from build123d import *

# Parameters (mm, degrees)
F1_DEPTH = 3
F2_R     = 1.25
F3_DEPTH = 10
F4_R     = 1
F5_DEPTH = 25
F6_W     = 1
F6_H     = 75
F7_DEPTH = 1


with BuildPart() as f1:
    # F0 (on Top) → F1 (new body)
    with BuildSketch(Plane.XY):
        with BuildLine():
            ThreePointArc((8.915987, -1.226854), (8.978972, -0.614863), (9, 0))
            ThreePointArc((9, 0), (8.978972, 0.614863), (8.915987, 1.226854))
            ThreePointArc((8.915987, 1.226854), (8.559509, 2.781153), (7.934312, 4.24814))
            ThreePointArc((7.934312, 4.24814), (7.281153, 5.290067), (6.492059, 6.233231))
            ThreePointArc((6.492059, 6.233231), (5.290067, 7.281153), (3.921999, 8.100489))
            ThreePointArc((3.921999, 8.100489), (2.781153, 8.559509), (1.588385, 8.858726))
            ThreePointArc((1.588385, 8.858726), (0, 9), (-1.588385, 8.858726))
            ThreePointArc((-1.588385, 8.858726), (-2.781153, 8.559509), (-3.921999, 8.100489))
            ThreePointArc((-3.921999, 8.100489), (-5.290067, 7.281153), (-6.492059, 6.233231))
            ThreePointArc((-6.492059, 6.233231), (-7.281153, 5.290067), (-7.934312, 4.24814))
            ThreePointArc((-7.934312, 4.24814), (-8.559509, 2.781153), (-8.915987, 1.226854))
            ThreePointArc((-8.915987, 1.226854), (-9, 0), (-8.915987, -1.226854))
            ThreePointArc((-8.915987, -1.226854), (-8.559509, -2.781153), (-7.934312, -4.24814))
            ThreePointArc((-7.934312, -4.24814), (-7.281153, -5.290067), (-6.492059, -6.233231))
            ThreePointArc((-6.492059, -6.233231), (-5.290067, -7.281153), (-3.921999, -8.100489))
            ThreePointArc((-3.921999, -8.100489), (-2.781153, -8.559509), (-1.588385, -8.858726))
            ThreePointArc((-1.588385, -8.858726), (0, -9), (1.588385, -8.858726))
            ThreePointArc((1.588385, -8.858726), (2.781153, -8.559509), (3.921999, -8.100489))
            ThreePointArc((3.921999, -8.100489), (5.290067, -7.281153), (6.492059, -6.233231))
            ThreePointArc((6.492059, -6.233231), (7.281153, -5.290067), (7.934312, -4.24814))
            ThreePointArc((7.934312, -4.24814), (8.559509, -2.781153), (8.915987, -1.226854))
        make_face()
        with BuildLine():
            ThreePointArc((7.934312, 4.24814), (8.559509, 2.781153), (8.915987, 1.226854))
            ThreePointArc((8.915987, 1.226854), (10.16558, 1.771623), (11.246167, 2.602639))
            Line((11.246167, 2.602639), (10.93715, 3.553695))
            Line((10.93715, 3.553695), (10.628133, 4.504752))
            ThreePointArc((10.628133, 4.504752), (9.265461, 4.541905), (7.934312, 4.24814))
        make_face()
        with BuildLine():
            ThreePointArc((11.246167, -2.602639), (10.16558, -1.771623), (8.915987, -1.226854))
            ThreePointArc((8.915987, -1.226854), (8.559509, -2.781153), (7.934312, -4.24814))
            ThreePointArc((7.934312, -4.24814), (9.265461, -4.541905), (10.628133, -4.504752))
            Line((10.628133, -4.504752), (10.93715, -3.553695))
            Line((10.93715, -3.553695), (11.246167, -2.602639))
        make_face()
        with BuildLine():
            ThreePointArc((3.921999, 8.100489), (5.290067, 7.281153), (6.492059, 6.233231))
            ThreePointArc((6.492059, 6.233231), (7.182793, 7.408451), (7.568547, 8.71591))
            Line((7.568547, 8.71591), (6.75953, 9.303695))
            Line((6.75953, 9.303695), (5.950513, 9.891481))
            ThreePointArc((5.950513, 9.891481), (4.826251, 9.120579), (3.921999, 8.100489))
        make_face()
        with BuildLine():
            ThreePointArc((7.568547, -8.71591), (7.182793, -7.408451), (6.492059, -6.233231))
            ThreePointArc((6.492059, -6.233231), (5.290067, -7.281153), (3.921999, -8.100489))
            ThreePointArc((3.921999, -8.100489), (4.826251, -9.120579), (5.950513, -9.891481))
            Line((5.950513, -9.891481), (6.75953, -9.303695))
            Line((6.75953, -9.303695), (7.568547, -8.71591))
        make_face()
        with BuildLine():
            ThreePointArc((-1.588385, 8.858726), (0, 9), (1.588385, 8.858726))
            ThreePointArc((1.588385, 8.858726), (1.456423, 10.215503), (1, 11.5))
            Line((1, 11.5), (0, 11.5))
            Line((0, 11.5), (-1, 11.5))
            ThreePointArc((-1, 11.5), (-1.456423, 10.215503), (-1.588385, 8.858726))
        make_face()
        with BuildLine():
            ThreePointArc((1, -11.5), (1.456423, -10.215503), (1.588385, -8.858726))
            ThreePointArc((1.588385, -8.858726), (0, -9), (-1.588385, -8.858726))
            ThreePointArc((-1.588385, -8.858726), (-1.456423, -10.215503), (-1, -11.5))
            Line((-1, -11.5), (0, -11.5))
            Line((0, -11.5), (1, -11.5))
        make_face()
        with BuildLine():
            ThreePointArc((-6.492059, 6.233231), (-5.290067, 7.281153), (-3.921999, 8.100489))
            ThreePointArc((-3.921999, 8.100489), (-4.826251, 9.120579), (-5.950513, 9.891481))
            Line((-5.950513, 9.891481), (-6.75953, 9.303695))
            Line((-6.75953, 9.303695), (-7.568547, 8.71591))
            ThreePointArc((-7.568547, 8.71591), (-7.182793, 7.408451), (-6.492059, 6.233231))
        make_face()
        with BuildLine():
            ThreePointArc((-5.950513, -9.891481), (-4.826251, -9.120579), (-3.921999, -8.100489))
            ThreePointArc((-3.921999, -8.100489), (-5.290067, -7.281153), (-6.492059, -6.233231))
            ThreePointArc((-6.492059, -6.233231), (-7.182793, -7.408451), (-7.568547, -8.71591))
            Line((-7.568547, -8.71591), (-6.75953, -9.303695))
            Line((-6.75953, -9.303695), (-5.950513, -9.891481))
        make_face()
        with BuildLine():
            ThreePointArc((-8.915987, 1.226854), (-8.559509, 2.781153), (-7.934312, 4.24814))
            ThreePointArc((-7.934312, 4.24814), (-9.265461, 4.541905), (-10.628133, 4.504752))
            Line((-10.628133, 4.504752), (-10.93715, 3.553695))
            Line((-10.93715, 3.553695), (-11.246167, 2.602639))
            ThreePointArc((-11.246167, 2.602639), (-10.16558, 1.771623), (-8.915987, 1.226854))
        make_face()
        with BuildLine():
            ThreePointArc((-10.628133, -4.504752), (-9.265461, -4.541905), (-7.934312, -4.24814))
            ThreePointArc((-7.934312, -4.24814), (-8.559509, -2.781153), (-8.915987, -1.226854))
            ThreePointArc((-8.915987, -1.226854), (-10.16558, -1.771623), (-11.246167, -2.602639))
            Line((-11.246167, -2.602639), (-10.93715, -3.553695))
            Line((-10.93715, -3.553695), (-10.628133, -4.504752))
        make_face()
    extrude(amount=F1_DEPTH)

    # F2 (on face) → F3 (join)
    with BuildSketch(Plane.XY.offset(3)):
        Circle(F2_R)
    extrude(amount=F3_DEPTH)

    # F4 (on face) → F5 (cut)
    with BuildSketch(Plane.XY.offset(13)):
        Circle(F4_R)
    extrude(amount=-F5_DEPTH, mode=Mode.SUBTRACT)

    # F6 (on face) → F7 (join)
    with BuildSketch(Plane.XY.offset(13)):
        with BuildLine():
            ThreePointArc((-1, 0.75), (-0.559017, 1.118034), (0, 1.25))
            Line((0, 1.25), (-1, 1.25))
            Line((-1, 1.25), (-1, 0.75))
        make_face()
        with Locations((-0.5, 38.75)):
            Rectangle(F6_W, F6_H)
        with Locations((0.5, 38.75)):
            Rectangle(F6_W, F6_H)
        with BuildLine():
            Line((1, 1.25), (0, 1.25))
            ThreePointArc((0, 1.25), (0.559017, 1.118034), (1, 0.75))
            Line((1, 0.75), (1, 1.25))
        make_face()
    extrude(amount=-F7_DEPTH)


solid = f1.part
Read the model definition and answer for the solid it produces. Units are mm, in the model's axes. A direction names the side the tool comes from. Round coordinates to 2 decimals unless told otherwise and drop trailing zeros. Write each loop counter-clockwise with the first axis right and the second up, starting at its lowest first coordinate (ties: lowest second). Pieces come first, ordered by that corner, then holes. Notation, with made-up numbers: (1, 27) - (52, 27) arc R16 cw to (52, 57) - close; hole circle Ø11 at (-29, -32.75). An arc over 180 degrees is marked (long way). Use a Markdown table: item, result.
(1) The part is cut by section C-C (z = 10.5). Write down the section's boundary in (x, y), then the cut area to 3 significant figures.
Reported:
| item | result |
|---|---|
| outline | circle Ø2.5 at (0, 0); hole circle Ø2 at (0, 0) |
| area | 1.77 mm2 |
(2) Each of these flat-tipped pins is pushed along its axis until it touches: pin 1 Ø0.8 at (y, z) = (24, 12.5) entering from +X; pin 2 Ø12 at (x, y) = (0, 37) entering from -Z; pin 3 Ø3 at (y, z) = (63, 9) entering from +X; pin 4 Ø6 at (x, z) = (7.5, 3.5) entering from +Y. Where does it stop, or does it pass through?
Reported:
| item | result |
|---|---|
| pin 1 | x = 1 |
| pin 2 | z = 12 |
| pin 3 | through |
| pin 4 | y = 9.89 |
(3) The mould has two halves that part along X. Classify faces 1 (the cylindrical face through (-7.175, -7.391, 1.479)), 2 (the cylindrical face through (10.18, -1.78, 1.48)), 3 (the cylindrical face through (-4.841, -9.133, 1.479)), 4 (the flat face through (0, 11.5, 1)): released by +X, released by -X, zero draft, split by the parting line, or undercut.
Reported:
| item | result |
|---|---|
| face 1 | released by -X |
| face 2 | released by +X |
| face 3 | undercut |
| face 4 | zero draft |
(4) The part is cut by section B-B (y = 45). Write down the section's boundary in (x, z), then the cut area to 3 significant figures.
Reported:
| item | result |
|---|---|
| outline | (-1, 12) - (1, 12) - (1, 13) - (-1, 13) - close |
| area | 2.00 mm2 |
(5) Which of the six approach directions +Z, -Z, +X, -X, +Y, -Y give full straight-line access (tool end or side, diameter ignored) to faces 5 (the cylindrical face through (-4.812, 9.108, 1.479)), 6 (the cylindrical face through (2.765, -8.565, 1.479)), 7 (the cylindrical face through (7.19, -7.43, 1.48))?
Reported:
| item | result |
|---|---|
| face 5 | +Z, -Z, +Y |
| face 6 | +Z, -Z, -Y |
| face 7 | +Z, -Z, +X |
(6) Straight lines are drawn through the part: line 1 along Y through (x, z) = (0, 7); line 2 along Z through (x, y) = (-2.25, -7); line 3 along Y through (x, z) = (-9.5, 2.25). For each, find the intervals that lie inside material, in ascending order. Write a range as [from, to].
Reported:
| item | result |
|---|---|
| line 1 | [-1.25, -1], [1, 1.25] |
| line 2 | [0, 3] |
| line 3 | [-4.56, -1.44], [1.44, 4.56] |
(7) The part is cut by section A-A (x = 0). Write down the section's boundary in (y, z), then the cut area to 3 significant figures.
Reported:
| item | result |
|---|---|
| outline | (-11.5, 0) - (-1, 0) - (-1, 13) - (-1.25, 13) - (-1.25, 3) - (-11.5, 3) - close; (1, 0) - (11.5, 0) - (11.5, 3) - (1.25, 3) - (1.25, 12) - (76.25, 12) - (76.25, 13) - (1, 13) - close |
| area | 143 mm2 |
